Model file for the job. Use its own axes, mm. A direction names the side the tool comes from. Round coordinates to 2 decimals unless told otherwise and drop trailing zeros. Order: outer loops, then holes, each group sorted by start corner. A loop starts at its lowest first (then second) coordinate and runs counter-clockwise, first axis right, second up. Notation, with made-up numbers: (48, -25.5) - (74, -25.5) arc R15 cw to (74, 0.5) - close; hole circle Ø1 at (-21, -17.5). An arc over 180 degrees is marked (long way). Write item = value, one per line.
```python
from build123d import *

# Parameters (mm, degrees)
F0_W      = 102
F0_H      = 54
F0_R      = 2.5
F1_DEPTH  = 2
F2_DEPTH  = 5
F3_DEPTH  = 38
F4_D      = 3
F4_DEPTH  = 5
F4_TIP    = 0.9012909285
F6_D      = 3
F6_DEPTH  = 20
F6_TIP    = 0.9012909285
F7_DEPTH  = 1
F8_R      = 5
F9_DEPTH  = 2
F10_W     = 11
F10_H     = 7
F10_R     = 2.1
F11_DEPTH = 2
F12_D     = 2
F12_DEPTH = 5
F12_TIP   = 0.600860619


with BuildPart() as f1:
    # F0 (on Top) → F1 (new body)
    with BuildSketch(Plane.XY):
        with BuildLine():
            Line((54, 37), (-54, 37))
            ThreePointArc((-54, 37), (-54.4644660941, 30.4644660941), (-61, 30))
            Line((-61, 30), (-61, -30))
            ThreePointArc((-61, -30), (-54.4644660941, -30.4644660941), (-54, -37))
            Line((-54, -37), (54, -37))
            ThreePointArc((54, -37), (54.4644660941, -30.4644660941), (61, -30))
            Line((61, -30), (61, 30))
            ThreePointArc((61, 30), (54.4644660941, 30.4644660941), (54, 37))
        make_face()
        Rectangle(F0_W, F0_H, mode=Mode.SUBTRACT)
        Rectangle(F0_W, F0_H)
        with Locations((14, -19.5)):
            Circle(F0_R, mode=Mode.SUBTRACT)
        with Locations((-36, 24)):
            Circle(F0_R, mode=Mode.SUBTRACT)
        with Locations((14, 8.5)):
            Circle(F0_R, mode=Mode.SUBTRACT)
    extrude(amount=F1_DEPTH)

    # F0 (on Top) → F2 (join)
    with BuildSketch(Plane.XY):
        with Locations((-36, 24)):
            Circle(F0_R)
        with Locations((14, 8.5)):
            Circle(F0_R)
        with Locations((14, -19.5)):
            Circle(F0_R)
    extrude(amount=F2_DEPTH)

    # F0 (on Top) → F3 (join)
    with BuildSketch(Plane.XY):
        with BuildLine():
            ThreePointArc((-61, 32), (-59.5355339059, 35.5355339059), (-56, 37))
            Line((-56, 37), (-54, 37))
            ThreePointArc((-54, 37), (-55.7639320225, 38.472135955), (-58, 39))
            ThreePointArc((-58, 39), (-61.5355339059, 37.5355339059), (-63, 34))
            ThreePointArc((-63, 34), (-62.472135955, 31.7639320225), (-61, 30))
            Line((-61, 30), (-61, 32))
        make_face()
        with BuildLine():
            ThreePointArc((58, 39), (55.7639320225, 38.472135955), (54, 37))
            Line((54, 37), (56, 37))
            ThreePointArc((56, 37), (59.5355339059, 35.5355339059), (61, 32))
            Line((61, 32), (61, 30))
            ThreePointArc((61, 30), (62.472135955, 31.7639320225), (63, 34))
            ThreePointArc((63, 34), (61.5355339059, 37.5355339059), (58, 39))
        make_face()
        with BuildLine():
            Line((56, 37), (54, 37))
            ThreePointArc((54, 37), (54.4644660941, 30.4644660941), (61, 30))
            Line((61, 30), (61, 32))
            ThreePointArc((61, 32), (59.5355339059, 35.5355339059), (56, 37))
        make_face()
        with BuildLine():
            Line((-54, 37), (-56, 37))
            ThreePointArc((-56, 37), (-59.5355339059, 35.5355339059), (-61, 32))
            Line((-61, 32), (-61, 30))
            ThreePointArc((-61, 30), (-54.4644660941, 30.4644660941), (-54, 37))
        make_face()
        with BuildLine():
            Line((-61, -30), (-61, 30))
            ThreePointArc((-61, 30), (-62.472135955, 31.7639320225), (-63, 34))
            Line((-63, 34), (-63, -34))
            ThreePointArc((-63, -34), (-62.472135955, -31.7639320225), (-61, -30))
        make_face()
        with BuildLine():
            ThreePointArc((-58, 39), (-55.7639320225, 38.472135955), (-54, 37))
            Line((-54, 37), (54, 37))
            ThreePointArc((54, 37), (55.7639320225, 38.472135955), (58, 39))
            Line((58, 39), (-58, 39))
        make_face()
        with BuildLine():
            ThreePointArc((63, 34), (62.472135955, 31.7639320225), (61, 30))
            Line((61, 30), (61, -30))
            ThreePointArc((61, -30), (62.472135955, -31.7639320225), (63, -34))
            Line((63, -34), (63, 34))
        make_face()
        with BuildLine():
            Line((61, -32), (61, -30))
            ThreePointArc((61, -30), (54.4644660941, -30.4644660941), (54, -37))
            Line((54, -37), (56, -37))
            ThreePointArc((56, -37), (59.5355339059, -35.5355339059), (61, -32))
        make_face()
        with BuildLine():
            ThreePointArc((-54, -37), (-54.4644660941, -30.4644660941), (-61, -30))
            Line((-61, -30), (-61, -32))
            ThreePointArc((-61, -32), (-59.5355339059, -35.5355339059), (-56, -37))
            Line((-56, -37), (-54, -37))
        make_face()
        with BuildLine():
            Line((-61, -32), (-61, -30))
            ThreePointArc((-61, -30), (-62.472135955, -31.7639320225), (-63, -34))
            ThreePointArc((-63, -34), (-61.5355339059, -37.5355339059), (-58, -39))
            ThreePointArc((-58, -39), (-55.7639320225, -38.472135955), (-54, -37))
            Line((-54, -37), (-56, -37))
            ThreePointArc((-56, -37), (-59.5355339059, -35.5355339059), (-61, -32))
        make_face()
        with BuildLine():
            Line((54, -37), (-54, -37))
            ThreePointArc((-54, -37), (-55.7639320225, -38.472135955), (-58, -39))
            Line((-58, -39), (58, -39))
            ThreePointArc((58, -39), (55.7639320225, -38.472135955), (54, -37))
        make_face()
        with BuildLine():
            ThreePointArc((63, -34), (62.472135955, -31.7639320225), (61, -30))
            Line((61, -30), (61, -32))
            ThreePointArc((61, -32), (59.5355339059, -35.5355339059), (56, -37))
            Line((56, -37), (54, -37))
            ThreePointArc((54, -37), (55.7639320225, -38.472135955), (58, -39))
            ThreePointArc((58, -39), (61.5355339059, -37.5355339059), (63, -34))
        make_face()
    extrude(amount=F3_DEPTH)

    # F4
    with Locations(Plane(origin=(0, 0, 0), x_dir=(1, 0, 0), z_dir=(0, 0, -1))):
        with Locations((56, 0), (-56, 0), (0, 32), (0, -32)):
            Hole(F4_D / 2, depth=F4_DEPTH)
            with Locations((0, 0, -(F4_DEPTH + F4_TIP / 2))):  # 118° drill point
                Cone(0, F4_D / 2, F4_TIP, mode=Mode.SUBTRACT)

    # F6
    with Locations(Plane.XY.offset(38)):
        with Locations((-58, 34), (58, 34), (58, -34), (-58, -34)):
            Hole(F6_D / 2, depth=F6_DEPTH)
            with Locations((0, 0, -(F6_DEPTH + F6_TIP / 2))):  # 118° drill point
                Cone(0, F6_D / 2, F6_TIP, mode=Mode.SUBTRACT)

    # F5 (on face) → F7 (cut)
    with BuildSketch(Plane.XY.offset(38)):
        with BuildLine():
            ThreePointArc((58, -39), (61.5355339059, -37.5355339059), (63, -34))
            Line((63, -34), (63, 34))
            ThreePointArc((63, 34), (61.5355339059, 37.5355339059), (58, 39))
            Line((58, 39), (-58, 39))
            ThreePointArc((-58, 39), (-61.5355339059, 37.5355339059), (-63, 34))
            Line((-63, 34), (-63, -34))
            ThreePointArc((-63, -34), (-61.5355339059, -37.5355339059), (-58, -39))
            Line((-58, -39), (58, -39))
        make_face()
        with BuildLine():
            ThreePointArc((58, 38), (60.8284271247, 36.8284271247), (62, 34))
            Line((62, 34), (62, -34))
            ThreePointArc((62, -34), (60.8284271247, -36.8284271247), (58, -38))
            Line((58, -38), (-58, -38))
            ThreePointArc((-58, -38), (-60.8284271247, -36.8284271247), (-62, -34))
            Line((-62, -34), (-62, 34))
            ThreePointArc((-62, 34), (-60.8284271247, 36.8284271247), (-58, 38))
            Line((-58, 38), (58, 38))
        make_face(mode=Mode.SUBTRACT)
    extrude(amount=-F7_DEPTH, mode=Mode.SUBTRACT)

    # F8 (on face) → F9 (cut, through all)
    with BuildSketch(Plane(origin=(-63, 0, 0), x_dir=(0, -1, 0), z_dir=(-1, 0, 0))):
        with Locations((18.5, 13)):
            Circle(F8_R)
    extrude(amount=-F9_DEPTH, mode=Mode.SUBTRACT)

    # F10 (on face) → F11 (cut, through all)
    with BuildSketch(Plane(origin=(0, 39, 0), x_dir=(-1, 0, 0), z_dir=(0, 1, 0))):
        with Locations((-22.5, 29.5)):
            Rectangle(F10_W, F10_H)
        with Locations((-7.5, 29.5)):
            Circle(F10_R)
    extrude(amount=-F11_DEPTH, mode=Mode.SUBTRACT)

    # F12
    with Locations(Plane(origin=(0, 0, 0), x_dir=(1, 0, 0), z_dir=(0, 0, -1))):
        with Locations((-36, -24), (14, -8.5), (14, 19.5)):
            Hole(F12_D / 2, depth=F12_DEPTH)
            with Locations((0, 0, -(F12_DEPTH + F12_TIP / 2))):  # 118° drill point
                Cone(0, F12_D / 2, F12_TIP, mode=Mode.SUBTRACT)


solid = f1.part
```
1) Cut at B-B (z = 24). Write the cut outline in (x, y), and give its area (3 significant figures).
Conclusion:
outline = (-63, -34) arc R5 ccw to (-58, -39) - (58, -39) arc R5 ccw to (63, -34) - (63, 34) arc R5 ccw to (58, 39) - (-58, 39) arc R5 ccw to (-63, 34) - close; hole (-61, -30) arc R5 cw to (-54, -37) - (54, -37) arc R5 cw to (61, -30) - (61, 30) arc R5 cw to (54, 37) - (-54, 37) arc R5 cw to (-61, 30) - close; hole circle Ø3 at (-58, -34); hole circle Ø3 at (-58, 34); hole circle Ø3 at (58, -34); hole circle Ø3 at (58, 34)
area = 977 mm^2
2) Flat gauge pins, fed straight in: pin 1 Ø6 at (x, y) = (-39.5, -4.5) entering from +Z; pin 2 Ø4 at (x, y) = (16, -19.5) entering from +Z; pin 3 Ø1.6 at (y, z) = (38, 30) entering from +X. Where does each tip first touch, or does it go through?
Conclusion:
pin_1 = 2
pin_2 = 5
pin_3 = 61.84
3) Cut at D-D (y = 4). Write the cut outline in (x, z), and give its area (3 significant figures).
Conclusion:
outline = (-63, 0) - (63, 0) - (63, 37) - (62, 37) - (62, 38) - (61, 38) - (61, 2) - (-61, 2) - (-61, 38) - (-62, 38) - (-62, 37) - (-63, 37) - close
area = 394 mm^2
4) Cut at A-A (z = 29.5). Write the cut outline in (x, y), and give its area (3 significant figures).
Conclusion:
outline = (-63, -34) arc R5 ccw to (-58, -39) - (58, -39) arc R5 ccw to (63, -34) - (63, 34) arc R5 ccw to (58, 39) - (28, 39) - (28, 37) - (54, 37) arc R5 ccw to (61, 30) - (61, -30) arc R5 ccw to (54, -37) - (-54, -37) arc R5 ccw to (-61, -30) - (-61, 30) arc R5 ccw to (-54, 37) - (5.4, 37) - (5.4, 39) - (-58, 39) arc R5 ccw to (-63, 34) - close; (9.6, 37) - (17, 37) - (17, 39) - (9.6, 39) - close; hole circle Ø3 at (-58, -34); hole circle Ø3 at (-58, 34); hole circle Ø3 at (58, -34); hole circle Ø3 at (58, 34)
area = 947 mm^2
5) Wall check: line 1 along X through (y, z) = (-34, 33.5); line 2 along Y through (x, z) = (-58, 32); line 3 along Y through (x, z) = (-36, 3). Give the ranges that are in metal, low to high.
Conclusion:
line_1 = -63 to -59.5, -56.5 to -53, 53 to 56.5, 59.5 to 63
line_2 = -39 to -35.5, -32.5 to -29, 29 to 32.5, 35.5 to 39
line_3 = -39 to -37, 21.5 to 23, 25 to 26.5, 37 to 39
6) Cut at C-C (x = 7.5). Write the cut outline in (y, z).
Conclusion:
outline = (-39, 0) - (39, 0) - (39, 27.4) - (37, 27.4) - (37, 2) - (-37, 2) - (-37, 38) - (-38, 38) - (-38, 37) - (-39, 37) - close; (37, 31.6) - (39, 31.6) - (39, 37) - (38, 37) - (38, 38) - (37, 38) - close
7) Mould opens along Y. For faces 5 (the face through (-60.859, 36.797, 37.507)), 6 (the face through (60.859, -36.797, 37.507)), 7 (the face through (1.2, 32.9, 1)) say: +Y half, -Y half, draft (parallel to the pull), parting line (faces both ways), or undercut.
Conclusion:
face_5 = +Y half
face_6 = -Y half
face_7 = undercut
8) 3-axis set-ups, long thin cutter, end or side, ignore diameter. For faces 1 (the face through (-62.01, -23.27, 14.5)), 2 (the face through (-60.797, -36.859, 37.507)), 3 (the face through (-1, -39, 18)), 4 (the face through (-59.386, -34.575, 27.86)): which of +Z, -Z, +X, -X, +Y, -Y reach the whole face in a straight line?
Conclusion:
face_1 = -X
face_2 = +Z, -X, -Y
face_3 = +Z, -Z, +X, -X, -Y
face_4 = +Z
